Autodesk Inventor part; units mm, degrees
ref_plane "YZ Plane" through (0, 0, 0) normal (1, 0, 0) x (0, 1, 0)
ref_plane "XZ Plane" through (0, 0, 0) normal (0, 1, 0) x (-1, 0, 0)
ref_plane "XY Plane" through (0, 0, 0) normal (0, 0, 1) x (1, 0, 0)
sketch "Sketch1" plane through (0, 0, 0) normal (0, 0, 1) x (1, 0, 0)
  line L0 (0, 0) -> (150, 0)
  line L1 (150, 0) -> (150, 350)
  line L2 (150, 350) -> (95.4045, 200)
  line L3 (0, 200) -> (95.4045, 200)
  line L4 (0, 0) -> (0, 200)
  line L5 (15, 0) -> (65, 0)
  line L6 (65, 0) -> (65, 5)
  line L7 (65, 5) -> (15, 5)
  line L8 (15, 5) -> (15, 0)
  line L9 (85, 0) -> (135, 0)
  line L10 (135, 0) -> (135, 5)
  line L11 (135, 5) -> (85, 5)
  line L12 (85, 5) -> (85, 0)
  line L13 (15, 200) -> (65, 200)
  line L14 (65, 200) -> (65, 195)
  line L15 (65, 195) -> (15, 195)
  line L16 (15, 195) -> (15, 200)
  line L17 (85, 200) -> (135, 200)
  line L18 (135, 200) -> (135, 195)
  line L19 (135, 195) -> (85, 195)
  line L20 (85, 195) -> (85, 200)
  point P0 (65, 200)
  point P1 (65, 0)
  point P2 (135, 0)
  dimension "d0" = 50
  dimension "d1" = 5
  dimension "d2" = 50
  dimension "d3" = 5
  dimension "d4" = 20
  dimension "d5" = 15
  dimension "d6" = 50
  dimension "d7" = 5
  dimension "d8" = 5
  dimension "d9" = 15
extrude "Extrusion1" add sketch "Sketch1" along normal blind 5 contours L4 L3 L16 L15 L14 L20 L19 L18 L17 L2 L1 L0 L10 L11 L12 L6 L7 L8
sketch "Sketch2" plane through (0, 0, 0) normal (0, 0, -1) x (-1, 0, 0)
  line L0 (-150, 0) -> (-150, 350)
  line L1 (-150, 160) -> (-145, 160)
  line L2 (-145, 160) -> (-145, 110)
  line L3 (-145, 110) -> (-150, 110)
  line L4 (-150, 110) -> (-150, 160)
  line L5 (-150, 80) -> (-145, 80)
  line L6 (-145, 80) -> (-145, 30)
  line L7 (-145, 30) -> (-150, 30)
  line L8 (-150, 30) -> (-150, 80)
  line L9 (-135, 0) -> (-150, 0)
  point P0 (0, 0)
  dimension "d12" = 5
  dimension "d13" = 50
  dimension "d14" = 5
  dimension "d15" = 50
  dimension "d16" = 30
  dimension "d17" = 30
extrude "Extrusion2" cut sketch "Sketch2" against normal blind 5
equation "\"d2\" = d0"
equation "\"d3\" = d1"
properties part number "Lateral"
Model file for the job. Use its own axes, mm. Give positions to 0.01 mm unless a question says otherwise; leave off trailing zeros. Order: outer loops, then holes, each group sorted by start corner. A loop starts at its lowest first (then second) coordinate and runs counter-clockwise, first axis right, second up.
1) Saw through at D-D, the plane x = 36. Write the cut outline in (y, z).
2) Saw through at C-C, the plane y = 118.5. Write the cut outline in (x, z).
3) Wall check: probe 1 along Y at (x, z) = (89, 2.4); probe 2 along X at (y, z) = (115, 4.6); probe 3 along X at (y, z) = (307.5, 3.55). Give the ranges that are in metal, low to high.
4) Saw through at A-A, the plane x = 127. Write the cut outline in (y, z).
5) Pin check, flat tip, straight feed: pin 1 (2.5 mm diameter, centred on x = 44.5, z = 1.5, fed in from +Y). Stop position of the tip, or through.
Computed:
1. outline: (5, 0) - (195, 0) - (195, 5) - (5, 5) - close
2. outline: (0, 0) - (145, 0) - (145, 5) - (0, 5) - close
3. probe 1: y = 5 to 195
3. probe 2: x = 0 to 145
3. probe 3: x = 134.53 to 150
4. outline: (5, 0) - (195, 0) - (195, 5) - (5, 5) - close; (200, 0) - (286.81, 0) - (286.81, 5) - (200, 5) - close
5. pin 1: stops at y = 195
